Geometry: final body of the model. Coordinates: model frame, mm. A direction names the side the tool comes from. Give positions to 0.01 mm unless a question says otherwise; leave off trailing zeros. Write each loop counter-clockwise with the first axis right and the second up, starting at its lowest first coordinate (ties: lowest second). Pieces come first, ordered by that corner, then holes. Notation, with made-up numbers: (-29.75, 43.25) -> (4.25, 43.25) arc R18 cw to (4.25, 47.25) -> close; hole circle Ø1 at (-28, 11.5). An arc over 180 degrees is marked (long way). Answer as a JSON object with one key per item and string values. Group by question number.
(1) Section query B-B on y = 10. Output: boundary loops of the cut face in (x, z).
(2) Set-up query: faces 1 (the face through (7.432, 11.755, 7.395)), 2 (the face through (8.8, 3, 18.8)), 3 (the face through (55, 1, 20)), 4 (the face through (65, 1, 20)). Return all of +Z, -Z, +X, -X, +Y, -Y with unobstructed straight access to the full face (end or side cutting, diameter ignored); none if empty.
(3) Material intervals for probe 1 along Z at (x, y) = (60, 0.7); probe 2 along Z at (x, y) = (19.5, 3.5); probe 3 along Y at (x, z) = (21.5, 1.75), sorted ascending.
(4) Section query A-A on z = 20. Output: boundary loops of the cut face in (x, y).
(5) Section query D-D on z = 6.5. Output: boundary loops of the cut face in (x, y), plus the area to 3 significant figures.
(6) Contact query for flat-ended pins moving along their axis: pin 1 Ø2.5 at (x, z) = (60, 20) entering from -Y; pin 2 Ø0.9 at (y, z) = (1, 19.5) entering from +X; pin 3 Ø0.9 at (y, z) = (1, 18) entering from -X; pin 4 Ø3 at (x, z) = (59.5, 20.5) entering from +Y. Output: stop coordinate, or through.
(7) Draft query along Y for faces 5 (the face through (39.05, 11.08, 7.4)), 6 (the face through (3.9, 6, 7)), 7 (the face through (15, 1, 20)), 8 (the face through (3.93, 12.88, 7.4)). Return one class per face: +Y half, -Y half, draft (parallel to the pull), parting line (faces both ways), or undercut.
(8) Section query C-C on x = 56. Output: boundary loops of the cut face in (y, z).
from build123d import *

# Parameters (mm, degrees)
F1_DEPTH = 15
F0_W     = 10
F0_H     = 3
F2_DEPTH = 25
F4_R     = 1.5
F3_R     = 1.5
F5_DEPTH = 5


with BuildPart() as f1:
    # F0 (on Top) → F1 (new body)
    with BuildSketch(Plane.XY):
        with BuildLine():
            Line((0, 4), (0, 0))
            Line((0, 0), (5, 0))
            Line((5, 0), (5, 3))
            Line((5, 3), (15, 3))
            Line((15, 3), (15, 0))
            Line((15, 0), (55, 0))
            Line((55, 0), (55, 3))
            Line((55, 3), (65, 3))
            Line((65, 3), (65, 0))
            Line((65, 0), (70, 0))
            Line((70, 0), (70, 4))
            Line((70, 4), (3.9, 4))
            Line((3.9, 4), (3.9, 7.923009))
            ThreePointArc((3.9, 7.923009), (7.496859, 11.792414), (12.645339, 12.976833))
            Line((12.645339, 12.976833), (66.200703, 9.12677))
            ThreePointArc((66.200703, 9.12677), (69.655888, 8.878378), (68.143409, 11.994852))
            Line((68.143409, 11.994852), (12.860452, 15.969111))
            ThreePointArc((12.860452, 15.969111), (3.824593, 12.784231), (0, 4))
        make_face()
    extrude(amount=F1_DEPTH)

    # F0 (on Top) → F2 (join)
    with BuildSketch(Plane.XY):
        with Locations((10, 1.5)):
            Rectangle(F0_W, F0_H)
        with Locations((60, 1.5)):
            Rectangle(F0_W, F0_H)
    extrude(amount=F2_DEPTH)

    # F4 (on face) + F3 (on face) → F5 (cut)
    with BuildSketch(Plane(origin=(0, 3, 0), x_dir=(-1, 0, 0), z_dir=(0, 1, 0))):
        with Locations((-60, 20)):
            Circle(F4_R)
    with BuildSketch(Plane(origin=(0, 3, 0), x_dir=(-1, 0, 0), z_dir=(0, 1, 0))):
        with Locations((-10, 20)):
            Circle(F3_R)
    extrude(amount=-F5_DEPTH, mode=Mode.SUBTRACT)


solid = f1.part
Answer list:
{
 "1": {"outline": "(1.61, 0) -> (5.29, 0) -> (5.29, 15) -> (1.61, 15) -> close; (54.05, 0) -> (70, 0) -> (70, 15) -> (54.05, 15) -> close"},
 "2": {"face 1": "+Z, -Z", "face 2": "+Z, +X, -X, +Y", "face 3": "+Z, +Y, -Y", "face 4": "+Z, +X, +Y, -Y"},
 "3": {"probe 1": "0 to 18.5, 21.5 to 25", "probe 2": "0 to 15", "probe 3": "0 to 4, 12.34 to 15.35"},
 "4": {"outline": "(5, 0) -> (8.5, 0) -> (8.5, 3) -> (5, 3) -> close; (11.5, 0) -> (15, 0) -> (15, 3) -> (11.5, 3) -> close; (55, 0) -> (58.5, 0) -> (58.5, 3) -> (55, 3) -> close; (61.5, 0) -> (65, 0) -> (65, 3) -> (61.5, 3) -> close"},
 "5": {"outline": "(0, 0) -> (70, 0) -> (70, 4) -> (3.9, 4) -> (3.9, 7.92) arc R9 cw to (12.65, 12.98) -> (66.2, 9.13) arc R2 ccw (long way) to (68.14, 11.99) -> (12.86, 15.97) arc R12 ccw to (0, 4) -> close", "area": "508 mm2"},
 "6": {"pin 1": "through", "pin 2": "x = 65", "pin 3": "x = 5", "pin 4": "y = 3"},
 "7": {"face 5": "undercut", "face 6": "undercut", "face 7": "draft", "face 8": "+Y half"},
 "8": {"outline": "(0, 0) -> (4, 0) -> (4, 15) -> (3, 15) -> (3, 25) -> (0, 25) -> close; (9.86, 0) -> (12.87, 0) -> (12.87, 15) -> (9.86, 15) -> close"}
}
